Could you check a few things on this model? Use its own coordinates, in mm. A direction names the side the tool comes from. Coordinates: 2 decimals unless noted, no trailing zeros. Loops run counter-clockwise (first coordinate to the right, second up) from the corner with the lowest first, then second, coordinate; pieces in that order, holes last.
1) Thinking about a two-plate mould opening in X: for faces 5 (the face through (-1, -12.5, 1)), 6 (the face through (-31.43, 0.18, -2.81)), 7 (the face through (25, 0, 20)), 8 (the face through (-25, 0, -27)), which applies, released by +X, released by -X, zero draft, split by the parting line, or undercut?
2) If I drill on line 1 along Y through (x, z) = (-6, 20); line 2 along X through (y, z) = (-5.5, 39.5); line 3 along Z through (x, y) = (-30, -3.25), over which ranges is the centre line in solid material (lowest first)?
3) Imagine slicing it at A-A on z = -4.5. Please give me the cut outline in (x, y), plus the area to 3 significant figures.
4) Imagine slicing it at D-D on x = 23. Please give me the cut outline in (y, z), plus the area to 3 significant figures.
5) Imagine slicing it at C-C on z = 18. Please give me the cut outline in (x, y).
6) Will these pins go through, and if not, where does the flat tip stop? P1, Ø8, axis at x = -5.78, y = 0, coming from the +Z side; P2, Ø12.5, axis at y = 5.5, z = 0, coming from the +X side; P3, Ø5, axis at x = 5.5, y = -9.5, coming from the -Z side; P4, Ø4, axis at y = -9.5, z = -28, coming from the +X side.
7) For faces 1 (the face through (-12.072, 1.982, -0.56)), 2 (the face through (-11, -6, -40)), 3 (the face through (-11, -6, 40)), 4 (the face through (2.5, 0, 0)), which set-ups out of +Z, -Z, +X, -X, +Y, -Y let a thin tool reach every point of the face, with its end or its side?
8) Imagine slicing it at B-B on y = 5. Please give me the cut outline in (x, z), plus the area to 3 significant figures.
```python
from build123d import *

# Parameters (mm, degrees)
F1_DEPTH       = 12.5
F3_D           = 13.2
F3_CBORE_D     = 19.25
F3_CBORE_DEPTH = 0
F5_D           = 13.2
F5_CBORE_D     = 19.25
F5_CBORE_DEPTH = 0
F6_W           = 45
F6_H           = 30
F7_DEPTH       = 30


with BuildPart() as f1:
    # F0 (on Front) → F1 (new body, symmetric)
    with BuildSketch(Plane.XZ):
        with BuildLine():
            Line((25, -25.5), (25, -40))
            Line((25, -40), (10.5, -40))
            ThreePointArc((10.5, -40), (25, -54.5), (39.5, -40))
            ThreePointArc((39.5, -40), (35.2530483272, -29.7469516728), (25, -25.5))
        make_face()
        with BuildLine():
            Line((10.5, -40), (25, -40))
            Line((25, -40), (25, -25.5))
            ThreePointArc((25, -25.5), (14.7469516728, -29.7469516728), (10.5, -40))
        make_face()
        with BuildLine():
            Line((-25, -40), (10.5, -40))
            ThreePointArc((10.5, -40), (14.7469516728, -29.7469516728), (25, -25.5))
            Line((25, -25.5), (25, 25.5))
            ThreePointArc((25, 25.5), (14.7469516728, 29.7469516728), (10.5, 40))
            Line((10.5, 40), (-25, 40))
            Line((-25, 40), (-25, 14.2162181315))
            ThreePointArc((-25, 14.2162181315), (-14.9640357801, 9.8540823977), (-10.8347666082, -0.279916916))
            ThreePointArc((-10.8347666082, -0.279916916), (-14.9640357801, -10.4139162298), (-25, -14.7760519636))
            Line((-25, -14.7760519636), (-25, -40))
        make_face()
        with BuildLine():
            ThreePointArc((10.5, 40), (14.7469516728, 29.7469516728), (25, 25.5))
            Line((25, 25.5), (25, 40))
            Line((25, 40), (10.5, 40))
        make_face()
        with BuildLine():
            Line((25, 40), (25, 25.5))
            ThreePointArc((25, 25.5), (35.2530483272, 29.7469516728), (39.5, 40))
            ThreePointArc((39.5, 40), (25, 54.5), (10.5, 40))
            Line((10.5, 40), (25, 40))
        make_face()
        with BuildLine():
            ThreePointArc((-25, 14.2162181315), (-39.8347666082, -0.279916916), (-25, -14.7760519636))
            Line((-25, -14.7760519636), (-25, 14.2162181315))
        make_face()
        with BuildLine():
            Line((-25, 14.2162181315), (-25, -14.7760519636))
            ThreePointArc((-25, -14.7760519636), (-14.9640357801, -10.4139162298), (-10.8347666082, -0.279916916))
            ThreePointArc((-10.8347666082, -0.279916916), (-14.9640357801, 9.8540823977), (-25, 14.2162181315))
        make_face()
    extrude(amount=F1_DEPTH, both=True)

    # F3 (through all)
    with Locations(Plane.XZ.offset(12.5)):
        with Locations((25, 40), (-25.3347666082, -0.279916916), (25, -40)):
            CounterBoreHole(F3_D / 2, F3_CBORE_D / 2, F3_CBORE_DEPTH)

    # F5 (through all)
    with Locations(Plane.XY.offset(40)):
        with Locations((-5.7768835686, 0)):
            CounterBoreHole(F5_D / 2, F5_CBORE_D / 2, F5_CBORE_DEPTH)

    # F6 (on face) → F7 (cut)
    with BuildSketch(Plane.XZ.offset(12.5)):
        with Locations((25, 0)):
            Rectangle(F6_W, F6_H)
    extrude(amount=-F7_DEPTH, mode=Mode.SUBTRACT)


solid = f1.part
```
Filled in:
1. face 5: zero draft
1. face 6: undercut
1. face 7: released by +X
1. face 8: released by -X
2. line 1: y = -12.5 to -6.6, 6.6 to 12.5
2. line 2: x = -25 to -9.43, -2.13 to 18.42, 31.58 to 39.49
2. line 3: z = -14.01 to -4.95, 4.39 to 13.45
3. outline: (-39.21, -12.5) - (-30.41, -12.5) - (-30.41, 12.5) - (-39.21, 12.5) - close; (-20.26, -12.5) - (2.5, -12.5) - (2.5, 12.5) - (-20.26, 12.5) - close; hole circle Ø13.2 at (-5.78, 0)
3. area: 652 mm2
4. outline: (-12.5, -54.36) - (12.5, -54.36) - (12.5, -46.29) - (-12.5, -46.29) - close; (-12.5, -33.71) - (12.5, -33.71) - (12.5, -15) - (-12.5, -15) - close; (-12.5, 15) - (12.5, 15) - (12.5, 33.71) - (-12.5, 33.71) - close; (-12.5, 46.29) - (12.5, 46.29) - (12.5, 54.36) - (-12.5, 54.36) - close
4. area: 1,340 mm2
5. outline: (-25, -12.5) - (25, -12.5) - (25, 12.5) - (-25, 12.5) - close; hole circle Ø13.2 at (-5.78, 0)
6. P1: passes through
6. P2: stops at x = 2.5
6. P3: stops at z = -40
6. P4: stops at x = 35.5
7. face 1: +Z, -Z
7. face 2: -Z, -X, +Y, -Y
7. face 3: +Z, -X, +Y, -Y
7. face 4: +X, +Y, -Y
8. outline: (-25, -40) - (-10.09, -40) - (-10.09, 40) - (-25, 40) - (-25, 14.22) arc R14.5 ccw (long way) to (-25, -14.78) - close; (-1.47, -40) - (10.5, -40) arc R14.5 ccw (long way) to (25, -25.5) - (25, -15) - (2.5, -15) - (2.5, 15) - (25, 15) - (25, 25.5) arc R14.5 ccw (long way) to (10.5, 40) - (-1.47, 40) - close; hole circle Ø13.2 at (-25.33, -0.28); hole circle Ø13.2 at (25, -40); hole circle Ø13.2 at (25, 40)
8. area: 3,560 mm2
